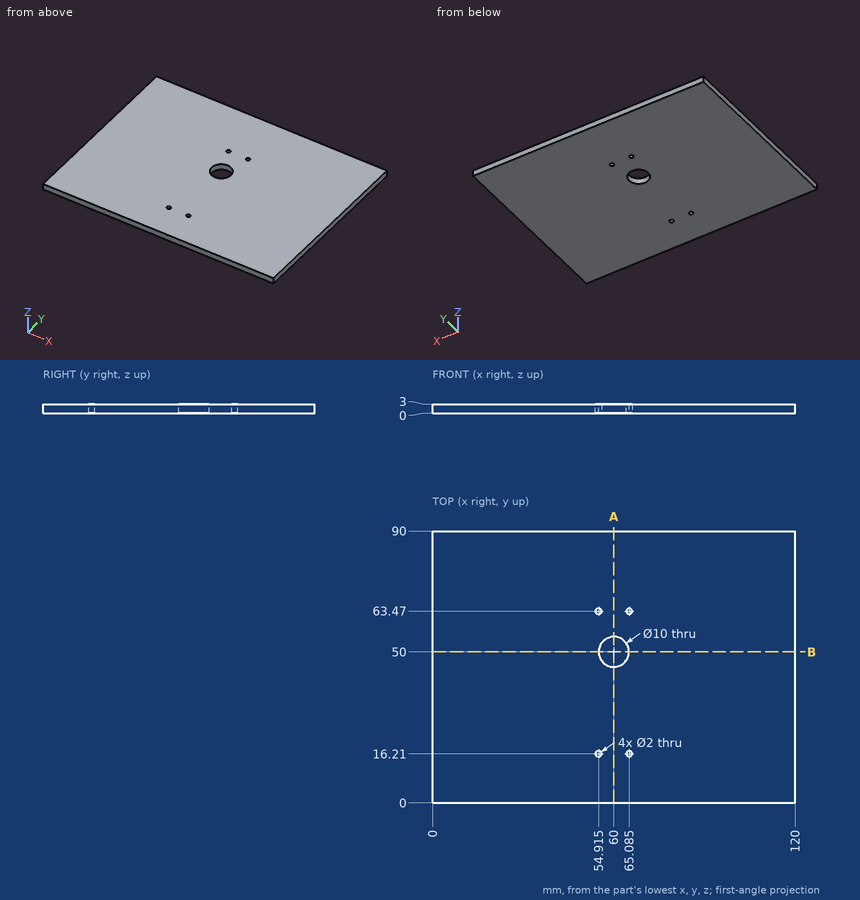
Check sheet for the drawn part. Datum: minimum x, y, z corner. Units: mm. Give positions to 0.01 mm unless a question says otherwise; leave off trailing zeros. Order: outer loops, then holes, each group sorted by start corner. A loop starts at its lowest first (then second) coordinate and runs counter-clockwise, first axis right, second up.
1. Depth check by flat-ended pin: pin 1 (5 mm diameter, centred on x = 75, y = 79, fed in from -Z); pin 2 (1.8 mm diameter, centred on x = 54.915, y = 63.47, fed in from +Z). Enter the tip coordinate at first touch or a pass-through.
Completed:
pin 1: stops at z = 0
pin 2: passes through
2. Scan lines: line 1 (X direction, y = 16.21, z = 2.25) (3 decimals); line 2 (Y direction, x = 60, z = 1.7); line 3 (Y direction, x = 57, z = 2.4). Record each from-to range of solid material in increasing order.
Completed:
line 1: x = 0 to 53.915, 55.915 to 64.085, 66.085 to 120
line 2: y = 0 to 45, 55 to 90
line 3: y = 0 to 46, 54 to 90
3. Sectioned sample at A-A (x = 60). Record the boundary of the cut face in (y, z).
Completed:
outline: (0, 0) - (45, 0) - (45, 3) - (0, 3) - close; (55, 0) - (90, 0) - (90, 3) - (55, 3) - close
4. Sectioned sample at B-B (y = 50). Record the boundary of the cut face in (x, z).
Completed:
outline: (0, 0) - (55, 0) - (55, 3) - (0, 3) - close; (65, 0) - (120, 0) - (120, 3) - (65, 3) - close
